For this review, take the finished solid that the model builds, in its own axes (mm). Give positions to 0.01 mm unless a question says otherwise; leave off trailing zeros. Order: outer loops, then holes, each group sorted by start corner. A loop starts at its lowest first (then second) coordinate and runs counter-clockwise, first axis right, second up.
Item 1: Consider section A-A (z = 0). Give the boundary of the cut face in (x, y) (3 decimals).
Item 2: For P1, Ø8, axis at x = 11.5, z = 29, coming from the -Y side; P2, Ø5, axis at y = 8, z = -25.5, coming from the -X side; P3, Ø2, axis at y = 42, z = 9.5, coming from the -X side, all flat-tipped, find the tip position at first contact; note any pin that passes through.
Item 3: Consider section B-B (y = 25). Give the boundary of the cut face in (x, z) (3 decimals).
Item 4: For probe 1 along X at (y, z) = (41, 0) (3 decimals); probe 2 along X at (y, z) = (28.5, 11.5) (3 decimals); probe 3 along Z at (x, y) = (-15.5, 21), list the stretches that pass through material, from the lowest coordinate up.
Item 5: Consider section C-C (x = -31). Give the boundary of the cut face in (y, z) (3 decimals), plus the area to 3 significant figures.
Item 6: The part is to be moulded in two halves that separate along X. For faces 1 (the flat face through (38.735, 32, 1)), 2 (the flat face through (20, 31, -38.735)), 3 (the cylindrical face through (-38.726, 31.306, -0.852)), 4 (the cylindrical face through (-34.714, 31.306, -7.709)), say which applies: released by +X, released by -X, zero draft, split by the parting line, or undercut.
```python
from build123d import *

# Parameters (mm, degrees)
SKETCH1_R                = 38.735
SKETCH1_R_2              = 35.56
BOSS_EXTRUDE1_DEPTH      = 63.5
BOSS_EXTRUDE2_REACH      = 109.398
BOSS_EXTRUDE2_END_RADIUS = 38.735
SKETCH2_W                = 77.47
SKETCH2_H                = 63.5


with BuildPart() as part:
    # Sketch1 → Boss-Extrude1 (new body)
    with BuildSketch(Plane(origin=(0, 0, 0), x_dir=(1, 0, 0), z_dir=(0, 1, 0))):
        with Locations(Location((0, 0, 0), (0, 0, 270))):
            Circle(SKETCH1_R)
        with Locations(Location((0, 0, 0), (0, 0, 270))):
            Circle(SKETCH1_R_2, mode=Mode.SUBTRACT)
    extrude(amount=BOSS_EXTRUDE1_DEPTH)

    # Boss-Extrude2: up to this cylinder (the profile starts outside it)
    boss_extrude2_end = Plane(origin=(0, 31.75, 0), z_dir=(0, -1, 0)) * Cylinder(BOSS_EXTRUDE2_END_RADIUS, 297.266, mode=Mode.PRIVATE)
    # Sketch2 → Boss-Extrude2 (add, up to the surface)
    with BuildSketch(Plane(origin=(38.735, 0, 0), x_dir=(0, 0, -1), z_dir=(1, 0, 0)), mode=Mode.PRIVATE) as boss_extrude2_sk1:
        with Locations((0, 31.75)):
            Rectangle(SKETCH2_W, SKETCH2_H)
    boss_extrude2_tool1 = extrude(boss_extrude2_sk1.sketch, amount=-BOSS_EXTRUDE2_REACH, mode=Mode.PRIVATE) - boss_extrude2_end
    add(boss_extrude2_tool1.solids().sort_by_distance((38.735, 31.75, 0))[0])
    add(boss_extrude2_tool1.solids().sort_by_distance((38.735, 31.75, 0))[1])


solid = part.part
```
Resolved:
1. outline: (-38.735, 0) - (-35.56, 0) - (-35.56, 63.5) - (-38.735, 63.5) - close; (35.56, 0) - (38.735, 0) - (38.735, 63.5) - (35.56, 63.5) - close
2. P1: passes through
2. P2: stops at x = -31.17
2. P3: stops at x = -37.79
3. outline: (0, -38.735) - (38.735, -38.735) - (38.735, 38.735) - (0, 38.735) arc R38.735 ccw to start; hole circle Ø71.12 at (0, 0)
4. probe 1: x = -38.735 to -35.56, 35.56 to 38.735
4. probe 2: x = -36.989 to -33.649, 33.649 to 38.735
4. probe 3: z = -35.5 to -32, 32 to 35.5
5. outline: (0, -23.225) - (63.5, -23.225) - (63.5, -17.422) - (0, -17.422) - close; (0, 17.422) - (63.5, 17.422) - (63.5, 23.225) - (0, 23.225) - close
5. area: 737 mm2
6. face 1: released by +X
6. face 2: zero draft
6. face 3: released by -X
6. face 4: undercut
